Part model, mm, in its own coordinate system. A direction names the side the tool comes from. Round coordinates to 2 decimals unless told otherwise and drop trailing zeros. Write each loop counter-clockwise with the first axis right and the second up, starting at its lowest first coordinate (ties: lowest second). Pieces come first, ordered by that corner, then holes.
1) Drill centre lines: L1, parallel to Z at x = 4.5, y = -4.25; L2, parallel to X at y = 4.25, z = 27.5; L3, parallel to Y at x = 0.5, z = 36.5. Where is each one in solid material? Low to high.
2) Pull direction Z, two halves, no side cores. Call faces 4 (the flat face through (5.3, -0.2, 84)), 5 (the flat face through (-4.309, -7.327, 94.158)), 6 (the conical face through (-7.649, -4.391, 91.316)), 7 (the flat face through (0, 0, 106)): +Z half, -Z half, draft (parallel to the pull), parting line (faces both ways), or undercut.
3) Flat gauge pins, fed straight in: pin 1 (2.5 mm diameter, centred on x = 5.5, y = -1, fed in from +Z); pin 2 (10 mm diameter, centred on y = -4.5, z = 73.5, fed in from +X); pin 3 (5 mm diameter, centred on x = 4.5, z = 27.5, fed in from +Y); pin 4 (1.4 mm diameter, centred on x = -4, y = 3.5, fed in from +Z). Where does each tip first touch, or does it go through?
4) Which spindle directions (+Z, -Z, +X, -X, +Y, -Y) get a long thin tool onto all of the face, cutting with end or side? Do faces 1 (the flat face through (4, -4, 91.2)), 2 (the flat face through (3.57, 3.5, 79.07)), 3 (the flat face through (0, 5.3, 84)). Say none if no direction does.
5) Saw through at A-A on z = 26. Write the cut outline in (x, y).
```python
from build123d import *

# Parameters (mm, degrees)
EXTRUDE_START       = 84
SKETCH_3_R          = 6
EXTRUDE_1_DEPTH     = 115.5
SKETCH_4_R          = 5
EXTRUDE_2_DEPTH     = 22
EXTRUDE_START_2     = 91.2
EXTRUDE_3_DEPTH     = 6
SKETCH_6_OUTSIDE_W  = 46.986
SKETCH_6_OUTSIDE_H  = 49.616
CUT_EXTRUDE_1_DEPTH = 10
CHAMFER_1_SIZE      = 0.6


with BuildPart() as part:
    # 草图3 → 凸台-拉伸1 (new body)
    with BuildSketch(Plane.XY.offset(EXTRUDE_START)):
        Circle(SKETCH_3_R)
    extrude(amount=-EXTRUDE_1_DEPTH)

    # 草图4 → 凸台-拉伸2 (add)
    with BuildSketch(Plane.XY.offset(84)):
        Circle(SKETCH_4_R)
    extrude(amount=EXTRUDE_2_DEPTH)

    # 草图5 → 凸台-拉伸3 (add)
    with BuildSketch(Plane.XY.offset(EXTRUDE_START_2)):
        Polygon((0, -9.814954576), (8.5, -4.907477288), (8.5, 4.907477288), (0, 9.814954576), (-8.5, 4.907477288), (-8.5, -4.907477288), align=None)
    extrude(amount=EXTRUDE_3_DEPTH)

    # 草图7 → 切除-旋转2 (revolve, cut)
    with BuildSketch(Plane(origin=(0, 0, 0), x_dir=(0, 0, -1), z_dir=(0, 1, 0))):
        Polygon((-97.2, 8.5), (-97.2, 18.742432258), (-91.2, 18.742432258), (-91.2, 8.5), (-94.2, 16.742432258), align=None)
    revolve(axis=Axis((0, 0, 84), (0, 0, 1)), mode=Mode.SUBTRACT)

    # 草图6 outside → 切除-拉伸1 (cut)
    with BuildSketch(Plane.XY.offset(84)):
        Rectangle(SKETCH_6_OUTSIDE_W, SKETCH_6_OUTSIDE_H)
        Polygon((0, -7.071067812), (7.071067812, 0), (0, 7.071067812), (-7.071067812, 0), align=None, mode=Mode.SUBTRACT)
    extrude(amount=-CUT_EXTRUDE_1_DEPTH, mode=Mode.SUBTRACT)

    # 倒角1
    chamfer_1_edges = [part.edges().sort_by_distance(p)[0] for p in [
        (-5, 0, 106),
    ]]
    chamfer(chamfer_1_edges, length=CHAMFER_1_SIZE)


solid = part.part
```
Completed:
1. L1: z = 91.2 to 97.2
1. L2: x = -4.24 to 4.24
1. L3: y = -5.98 to 5.98
2. face 4: undercut
2. face 5: draft
2. face 6: -Z half
2. face 7: +Z half
3. pin 1: stops at z = 106
3. pin 2: stops at x = 6
3. pin 3: stops at y = 5.66
3. pin 4: stops at z = 105.78
4. face 1: none
4. face 2: +X, +Y
4. face 3: +Y
5. outline: circle Ø12 at (0, 0)
